```python
from build123d import *

# Parameters (mm, degrees)
SKETCH1_R            = 60
SKETCH1_R_2          = 45
BOSS_EXTRUDE3_DEPTH  = 4
SKETCH9_R            = 49
SKETCH9_R_2          = 45
BOSS_EXTRUDE5_DEPTH  = 54
SKETCH10_W           = 8
SKETCH10_H           = 40
SKETCH10_W_2         = 15
SKETCH10_H_2         = 8
BOSS_EXTRUDE6_DEPTH  = 13
SKETCH12_W           = 10
SKETCH12_H           = 25
CUT_EXTRUDE1_DEPTH   = 8
SKETCH13_R           = 5
CUT_EXTRUDE2_DEPTH   = 110.729496946
SKETCH14_R           = 1.4
CUT_EXTRUDE3_DEPTH   = 7.2
BOSS_EXTRUDE10_DEPTH = 4
SKETCH18_R           = 2.5
CUT_EXTRUDE4_DEPTH   = 101.578327739


with BuildPart() as part:
    # Sketch1 → Boss-Extrude3 (new body)
    with BuildSketch(Plane(origin=(0, 0, 0), x_dir=(1, 0, 0), z_dir=(0, 1, 0))):
        with Locations(Location((0, 0, 0), (0, 0, 270))):
            Circle(SKETCH1_R)
        with Locations(Location((0, 0, 0), (0, 0, 270))):
            Circle(SKETCH1_R_2, mode=Mode.SUBTRACT)
    extrude(amount=BOSS_EXTRUDE3_DEPTH)

    # Sketch9 → Boss-Extrude5 (add)
    with BuildSketch(Plane(origin=(0, 4, 0), x_dir=(1, 0, 0), z_dir=(0, 1, 0))):
        with Locations(Location((0, 0, 0), (0, 0, 270))):
            Circle(SKETCH9_R)
        with Locations(Location((0, 0, 0), (0, 0, 270))):
            Circle(SKETCH9_R_2, mode=Mode.SUBTRACT)
    extrude(amount=BOSS_EXTRUDE5_DEPTH)

    # Sketch10 → Boss-Extrude6 (add, symmetric)
    with BuildSketch(Plane.XY):
        with Locations((15.25, 20)):
            Rectangle(SKETCH10_W, SKETCH10_H)
        with Locations((-39.25, 44)):
            Rectangle(SKETCH10_W_2, SKETCH10_H_2)
    extrude(amount=BOSS_EXTRUDE6_DEPTH, both=True)


with BuildPart() as boss_extrude6_piece_1:
    # of the separate pieces the step leaves, piece 1, a body of its own (boss_extrude6_pieces)
    add(part.part.solids().sort_by_distance((0, 0, 60))[0])

    # Sketch13 → Cut-Extrude2 (cut, through all)
    with BuildSketch(Plane.ZY.offset(-11.25)):
        with Locations((0, 19)):
            Circle(SKETCH13_R)
    extrude(amount=-CUT_EXTRUDE2_DEPTH, mode=Mode.SUBTRACT)



with BuildPart() as boss_extrude6_piece_2:
    # of the separate pieces the step leaves, piece 2, a body of its own (boss_extrude6_pieces)
    add(part.part.solids().sort_by_distance((11.25, 0, -13))[0])

    # Sketch12 → Cut-Extrude1 (cut)
    with BuildSketch(Plane.ZY.offset(-11.25)):
        with Locations((0, 17.5)):
            Rectangle(SKETCH12_W, SKETCH12_H)
    extrude(amount=-CUT_EXTRUDE1_DEPTH, mode=Mode.SUBTRACT)

    # Sketch14 → Cut-Extrude3 (cut)
    with BuildSketch(Plane.XZ):
        with Locations((-34, -7.797761416)):
            Circle(SKETCH14_R)
        with Locations(Location((14, -7.797761416, 0), (0, 0, 270))):
            Circle(SKETCH14_R)
        with Locations(Location((14, 7.797761416, 0), (0, 0, 90))):
            Circle(SKETCH14_R)
        with Locations((-34, 7.797761416)):
            Circle(SKETCH14_R)
    extrude(amount=-CUT_EXTRUDE3_DEPTH, mode=Mode.SUBTRACT)


with BuildPart() as boss_extrude6_piece_1_1:
    add(boss_extrude6_piece_1.part)

    add(boss_extrude6_piece_2.part)  # Boss-Extrude10 merges Boss-Extrude6 piece 2
    # Sketch15 → Boss-Extrude10 (add)
    with BuildSketch(Plane.XZ):
        with BuildLine():
            Line((25.249838503, 37.248431585), (11.25, 13))
            Line((11.25, 13), (11.25, -13))
            Line((11.25, -13), (25.249838503, -37.248431585))
            ThreePointArc((25.249838503, -37.248431585), (39.757029144, -21.080290171), (45, 0))
            ThreePointArc((45, 0), (39.757029144, 21.080290171), (25.249838503, 37.248431585))
        make_face()
        with BuildLine():
            Line((24.25, -21.516660498), (24.25, 21.516660498))
            Line((24.25, 21.516660498), (27.167270196, 26.569520697))
            ThreePointArc((27.167270196, 26.569520697), (38, 0), (27.167270196, -26.569520697))
            Line((27.167270196, -26.569520697), (24.25, -21.516660498))
        make_face(mode=Mode.SUBTRACT)
    extrude(amount=-BOSS_EXTRUDE10_DEPTH)

    # Sketch18 → Cut-Extrude4 (cut, through all)
    with BuildSketch(Plane(origin=(0, 4, 0), x_dir=(1, 0, 0), z_dir=(0, 1, 0))):
        with Locations(Location((46.451404387, 29.449397795, 0), (0, 0, 270))):
            Circle(SKETCH18_R)
        with Locations(Location((29.449397795, -46.451404387, 0), (0, 0, 270))):
            Circle(SKETCH18_R)
        with Locations(Location((-46.451404387, -29.449397795, 0), (0, 0, 270))):
            Circle(SKETCH18_R)
        with Locations(Location((-29.449397795, 46.451404387, 0), (0, 0, 270))):
            Circle(SKETCH18_R)
    extrude(amount=-CUT_EXTRUDE4_DEPTH, mode=Mode.SUBTRACT)


solid = boss_extrude6_piece_1_1.part
```
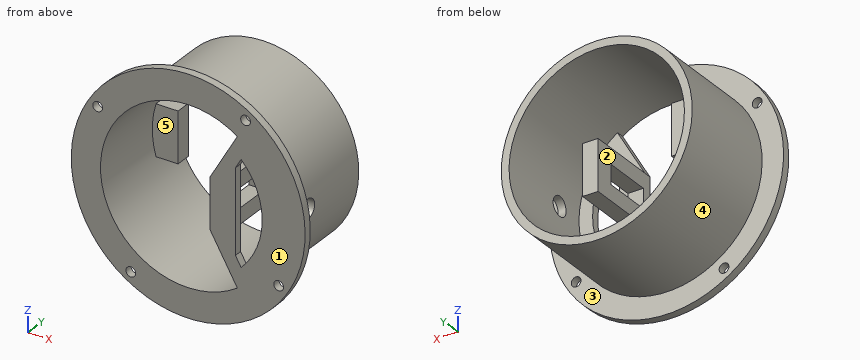
Could you check a few things on this model? Use its own coordinates, in mm. Face numbers are marked on the shaded views. A direction names the side the tool comes from. Round coordinates to 2 decimals unless told otherwise and drop trailing zeros. Loops run counter-clockwise (first coordinate to the right, second up) from the corner with the lowest first, then second, coordinate; pieces in that order, holes last. Notation, with made-up numbers: (76, 88.25) - (123, 88.25) arc R17 ccw to (123, 112.25) - close; hole circle Ø3 at (54.25, 46.5). An arc over 180 degrees is marked (long way). Answer as CSV lines item,"result".
1. On a 3-axis mill with a long thin cutter (end or side, diameter ignored), from which of +Z, -Z, +X, -X, +Y, -Y can I reach the whole of each face in a straight line? I mean the marked faces 1 and 2. Say none if no direction works.
Filled in:
face 1,"+Z, -Z, +X, -X, -Y"
face 2,"+Y, -Y"
2. We'd pull the mould along X, two halves only. Please class the marked faces 3, 4 and 5: +X half, -X half, draft (parallel to the pull), parting line (faces both ways), or undercut.
Filled in:
face 3,"draft"
face 4,"parting line"
face 5,"undercut"
3. Please list where these lines run through material, in increasing order: line 1 along X through (y, z) = (37.5, -1.5) (3 decimals); line 2 along Z through (x, y) = (25, 3); line 3 along Z through (x, y) = (29, 15). Write a range as [from, to].
Filled in:
line 1,"x = [-48.977, -44.975], [11.25, 19.25], [44.975, 48.977]"
line 2,"z = [-54.54, -37.42], [-36.82, -22.82], [22.82, 36.82], [37.42, 54.54]"
line 3,"z = [-39.5, -34.41], [34.41, 39.5]"
4. I want a section at B-B on y = 11.5. List the corners of the cut face in (x, z) for me, then the cut area to 3 significant figures.
Filled in:
outline,"circle Ø98 at (0, 0); (11.25, -13) - (19.25, -13) - (19.25, -5) - (11.25, -5) - close; (11.25, 5) - (19.25, 5) - (19.25, 13) - (11.25, 13) - close; hole circle Ø90 at (0, 0)"
area,"1,310 mm^2"
5. I want a section at D-D on x = -41. List the corners of the cut face in (y, z) for me.
Filled in:
outline,"(0, -43.81) - (4, -43.81) - (4, -26.83) - (58, -26.83) - (58, -18.55) - (0, -18.55) - close; (0, 18.55) - (58, 18.55) - (58, 26.83) - (4, 26.83) - (4, 43.81) - (0, 43.81) - close; (40, -13) - (48, -13) - (48, 13) - (40, 13) - close"
6. I want a section at C-C on x = 0. List the corners of the cut face in (y, z) for me.
Filled in:
outline,"(0, -60) - (4, -60) - (4, -49) - (58, -49) - (58, -45) - (0, -45) - close; (0, 45) - (58, 45) - (58, 49) - (4, 49) - (4, 60) - (0, 60) - close"
7. For pin 1 Ø8 at (x, z) = (-29.45, -46.45) entering from +Y; pin 2 Ø3 at (y, z) = (43.5, 44) entering from +X; pin 3 Ø12 at (y, z) = (40, 12.5) entering from -X, each with a flat end and sliding along its axis, tell me the tip position at first contact or that it passes through.
Filled in:
pin 1,"stops at y = 4"
pin 2,"stops at x = 24.39"
pin 3,"stops at x = -48.57"
8. I want a section at A-A on z = 0. Count the separate pieces of the cut face and the enclosed holes in it, then the cut area to 3 significant figures.
Filled in:
separate pieces,"5"
enclosed holes,"0"
area,"786 mm^2"
